Job drawing, mm, ordinate dimensions from the low corner. One solid piece. Give positions to 0.01 mm unless a question says otherwise; leave off trailing zeros. Order: outer loops, then holes, each group sorted by start corner. A loop starts at its lowest first (then second) coordinate and runs counter-clockwise, first axis right, second up.
1. Slice it at A-A on y = 26. List the corners of the cut face in (x, z).
2. Drop flat-ended pins along their axis: pin 1 Ø1.5 at (y, z) = (31, 7) entering from +X; pin 2 Ø12 at (x, y) = (33, 7.5) entering from -Z; pin 3 Ø10 at (x, z) = (44, 10.5) entering from +Y; pin 4 Ø2.5 at (x, y) = (3.5, 28) entering from +Z. Give the stop position or say it passes through.
3. Probe line 1 (Y direction, x = 33, z = 21); line 2 (Z direction, x = 31.5, y = 9); line 3 (X direction, y = 25.5, z = 19.75) (3 decimals). List the from-to ranges inside material, lowest first.
4. Mould opens along Y. For the marked faces 1, 2 and 3 say: +Y half, -Y half, draft (parallel to the pull), parting line (faces both ways), or undercut.
5. Slice it at B-B on x = 33. List the corners of the cut face in (y, z), and give its area (3 significant figures).
6. Slice it at C-C on z = 20.75. List the corners of the cut face in (x, y), and give its area (3 significant figures).
7. Slice it at D-D on y = 48. List the corners of the cut face in (x, z).
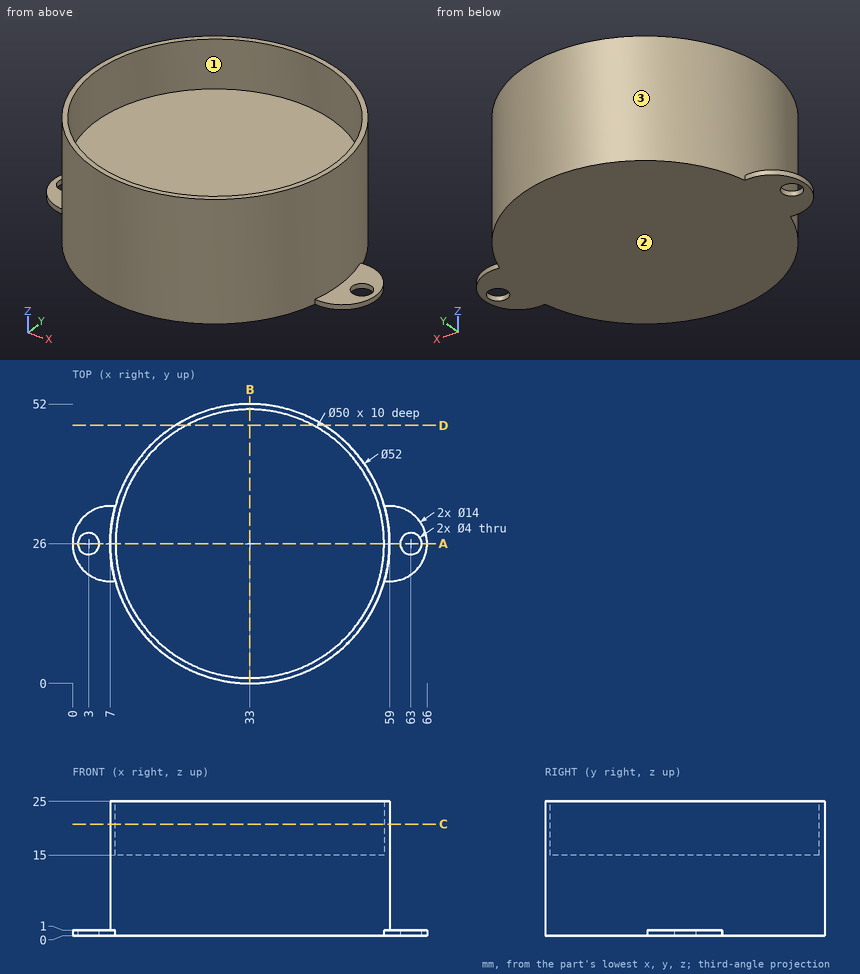
Data:
1. outline: (0, 0) - (1, 0) - (1, 1) - (0, 1) - close; (5, 0) - (61, 0) - (61, 1) - (59, 1) - (59, 25) - (58, 25) - (58, 15) - (8, 15) - (8, 25) - (7, 25) - (7, 1) - (5, 1) - close; (65, 0) - (66, 0) - (66, 1) - (65, 1) - close
2. pin 1: stops at x = 58.65
2. pin 2: stops at z = 0
2. pin 3: stops at y = 51.3
2. pin 4: stops at z = 1
3. line 1: y = 0 to 1, 51 to 52
3. line 2: z = 0 to 15
3. line 3: x = 7.005 to 8.005, 57.995 to 58.995
4. face 1: undercut
4. face 2: draft
4. face 3: parting line
5. outline: (0, 0) - (52, 0) - (52, 25) - (51, 25) - (51, 15) - (1, 15) - (1, 25) - (0, 25) - close
5. area: 800 mm2
6. outline: circle Ø52 at (33, 26); hole circle Ø50 at (33, 26)
6. area: 160 mm2
7. outline: (19.14, 0) - (46.86, 0) - (46.86, 25) - (44.87, 25) - (44.87, 15) - (21.13, 15) - (21.13, 25) - (19.14, 25) - close
